The listing builds one solid part. Answer for the finished solid, in the listing's coordinates (mm). Coordinates: 2 decimals unless noted, no trailing zeros. Order: outer loops, then holes, each group sorted by start corner. A loop starts at its lowest first (then second) coordinate and runs counter-clockwise, first axis right, second up. Notation, with made-up numbers: (18, -6.75) -> (45, -6.75) arc R10 ccw to (45, 3.25) -> close; hole circle Ø8 at (-24, 11). An arc over 180 degrees is marked (long way). Answer in a Markdown table with one row per item.
Autodesk Inventor part; units mm, degrees
ref_plane "Work Plane1" through (0, 2.14, 0) normal (0, 0, -1) x (0, 1, 0)
ref_plane "YZ Plane" through (0, 0, 0) normal (1, 0, 0) x (0, 1, 0)
ref_plane "XZ Plane" through (0, 0, 0) normal (0, 1, 0) x (-1, 0, 0)
sketch "Sketch5" plane through (0, 0, 0) normal (0, 1, 0) x (-1, 0, 0)
  line L0 (-1.225, -1.1) -> (1.225, -1.1)
  line L1 (1.225, -1.1) -> (1.225, 1.1)
  line L2 (1.225, 1.1) -> (-1.225, 1.1)
  line L3 (-1.225, 1.1) -> (-1.225, -1.1)
  line L4 (-1.225, -1.1) -> (1.225, 1.1) construction
  line L5 (1.225, -1.1) -> (-1.225, 1.1) construction
  line L6 (1.225, 1.1) -> (1.075, 1.27)
  line L7 (1.075, 1.27) -> (-1.075, 1.27)
  line L8 (-1.075, 1.27) -> (-1.225, 1.1)
  line L9 (0, 1.1) -> (0, -1.1) construction
  line L10 (1.225, 0) -> (-1.225, 0) construction
  line L11 (1.225, -1.1) -> (1.075, -1.27)
  line L12 (1.075, -1.27) -> (-1.075, -1.27)
  line L13 (-1.075, -1.27) -> (-1.225, -1.1)
  point P0 (0, 0)
  dimension "d33" = 2.2
  dimension "d34" = 2.45
  dimension "d36" = 0.15
  dimension "d37" = 2.54
extrude "Extrusion4" add sketch "Sketch5" along normal blind 2.54
sketch "Sketch6" plane through (-1.075, 0, 1.27) normal (0, 0, 1) x (1, 0, 0)
  line L0 (0, 2.54) -> (2.15, 2.54)
  line L1 (2.15, 2.14) -> (0, 2.14)
  line L2 (0, 2.14) -> (0, 2.54)
  line L3 (0, 2.54) -> (2.15, 2.54)
  line L4 (2.15, 2.54) -> (2.15, 2.14)
  line L5 (2.15, 2.14) -> (0, 2.54) construction
  line L6 (0, 2.14) -> (2.15, 2.54) construction
  line L7 (1.075, 0) -> (1.075, 2.54) construction
  point P0 (1.075, 2.34)
  dimension "d40" = 2.15
  dimension "d41" = 0.4
extrude "Extrusion5" cut sketch "Sketch6" against normal through all
chamfer "Chamfer3" distance 0.1 angle 45 2 edges at (-1.075, 2.14, 0) (1.075, 2.14, 0)
chamfer "Chamfer4" distance 0.03 angle 45 2 edges at (1.075, 2.54, 0) (-1.075, 2.54, 0)
sketch "Sketch7" plane through (-0.975, 2.14, 1.27) normal (0, 1, 0) x (1, 0, 0)
  circle A0 centre (0.975, 1.27) radius 0.3
  dimension "d50" = 0.6
extrude "Extrusion6" add sketch "Sketch7" along normal blind 3.6 and the other way blind 7.2
chamfer "Chamfer5" distance 0.2 angle 45 2 edges at (-0.3, 5.74, 0) (-0.3, -5.06, 0)
ref_plane "Work Plane1" through (0, 2.14, 0) normal (0, 0, -1) x (0, 1, 0)
sketch "Sketch8" plane through (0, 2.14, 0) normal (0, 0, -1) x (0, 1, 0)
  line L0 (0, -0.3) -> (3.4, -0.3)
  line L1 (1.975, -0.75) -> (1.975, 0)
  line L2 (3.4, 0) -> (3.4, -0.3)
  line L3 (0, 0.3) -> (0, -0.3)
  line L4 (3.4, -0.3) -> (3.4, 0.3)
  line L5 (3.6, 0.1) -> (3.6, -0.1) construction
  line L6 (3.6, 0) -> (0, 0) construction
  line L7 (-9.36, 0) -> (5.76, 0) construction
  line L8 (0.4, -1.225) -> (0.4, -1.105) construction
  line L9 (3.4, -0.3) -> (3.4, 0.3)
  line L10 (3.4, 0) -> (1.975, 0)
  line L11 (3.4, -0.3) -> (2.9466, -0.3) construction
  line L12 (2.9466, -0.3) -> (2.3806, -0.5247) construction
  line L13 (2.3806, -0.5247) -> (1.975, -0.75) construction
  spline S0 degree 3 poles (3.4, -0.3) (2.9466, -0.3) (2.3806, -0.5247) (1.975, -0.75) knots 1 1 1 1 2 2 2 2
  point P0 (-2.14, 0)
  point P1 (1.975, -0.3)
  dimension "d59" = 1.575
  dimension "d61" = 0.75
revolve "Revolution1" add sketch "Sketch8" angle 360 about axis through (0, 2.14, 0) along (0, 1, 0) contours L0 S0 L1
properties part number "pins"
(1) A flat-ended cylindrical pin translates along its axis: pin 1 (1 mm diameter, centred on x = 0.5, z = -0.5, fed in from +Y). Find the tip coordinate at first contact, or state that the pin passes through.
Check values:
| item | result |
|---|---|
| pin 1 | y = 5.63 |
(2) A cutting plane is placed at A-A, the plane z = -0.9. Determine the outline of the cut face in (x, y) (3 decimals).
Check values:
| item | result |
|---|---|
| outline | (-1.225, 0) -> (1.225, 0) -> (1.225, 2.54) -> (1.105, 2.54) -> (1.075, 2.51) -> (1.075, 2.24) -> (0.975, 2.14) -> (-0.975, 2.14) -> (-1.075, 2.24) -> (-1.075, 2.51) -> (-1.105, 2.54) -> (-1.225, 2.54) -> close |
(3) A cutting plane is placed at B-B, the plane y = 3. Determine the outline of the cut face in (x, z), then the cut area to 3 significant figures.
Check values:
| item | result |
|---|---|
| outline | circle Ø0.6 at (0, 0) |
| area | 0.283 mm² |
(4) Find the intervals of material crossed by line 1 along Y through (x, z) = (0.25, -1); line 2 along Y through (x, z) = (-0.6, 0.15) (3 decimals); line 3 along X through (y, z) = (-1, 0.1), in increasing order. Write a range as from..to.
Check values:
| item | result |
|---|---|
| line 1 | 0..2.14 |
| line 2 | 0..2.14, 4.115..4.372 |
| line 3 | -0.28..0.28 |
